from build123d import *

# Parameters (mm, degrees)
SKETCH2_R            = 65
SKETCH2_R_2          = 36
RING_EXTRUSION_DEPTH = 2
GROOVES_DEPTH        = 1
CIRPATTERN2_COUNT    = 12
FILLET3_R            = 0.5


with BuildPart() as part:
    # Sketch2 → ring extrusion (new body)
    with BuildSketch(Plane(origin=(0, 0, 0), x_dir=(1, 0, 0), z_dir=(0, 1, 0))):
        with Locations(Location((0, 0, 0), (0, 0, 270))):
            Circle(SKETCH2_R)
        with Locations(Location((0, 0, 0), (0, 0, 270))):
            Circle(SKETCH2_R_2, mode=Mode.SUBTRACT)
    extrude(amount=RING_EXTRUSION_DEPTH)

    # Sketch5 → grooves (cut)
    with BuildSketch(Plane(origin=(0, 2, 0), x_dir=(1, 0, 0), z_dir=(0, 1, 0))):
        with BuildLine():
            Line((-43, 38.6), (7, 38.6))
            ThreePointArc((7, 38.6), (7.6, 38), (7, 37.4))
            Line((7, 37.4), (-43, 37.4))
            ThreePointArc((-43, 37.4), (-43.6, 38), (-43, 38.6))
        make_face()
    grooves = extrude(amount=-GROOVES_DEPTH, mode=Mode.SUBTRACT)

    # CirPattern2: grooves ×12 about axis
    cirpattern2_axis = Axis((0, 0, 0), (0, 1, 0))
    for i in range(1, CIRPATTERN2_COUNT):
        add(grooves.rotate(cirpattern2_axis, i * 360 / CIRPATTERN2_COUNT), mode=Mode.SUBTRACT)

    # Fillet3
    fillet3_edges = [part.edges().sort_by_distance(p)[0] for p in [
        (0, 0, -65),
        (0, 2, -65),
        (0, 0, -36),
        (0, 2, -36),
    ]]
    fillet(fillet3_edges, radius=FILLET3_R)


solid = part.part
For this review, take the finished solid that the model builds, in its own axes (mm). A direction names the side the tool comes from. Round coordinates to 2 decimals unless told otherwise and drop trailing zeros. One line per item, written item: value. Start each with the question number.
Item 1: Clearance check with flat-ended pins moving along their axes: pin 1 Ø0.5 at (y, z) = (1.5, -28.5) entering from +X; pin 2 Ø1 at (y, z) = (1.5, 23.5) entering from +X; pin 3 Ø1.1 at (y, z) = (1.5, 10.5) entering from -X. State where each tip first meets the part, or that it passes through.
Item 2: The part is to be moulded in two halves that separate along Z. For faces 1 (the cylindrical face through (19.52, 0.99, 62)), 2 (the flat face through (-42, 2, -1)), 3 (the flat face through (34, 1, 24)), say which applies: +Z half, -Z half, draft (parallel to the pull), parting line (faces both ways), or undercut.
Item 3: For L1, parallel to Z at x = 50.5, y = 1.6; L2, parallel to X at y = 1.55, z = 49.5; L3, parallel to Z at x = 12, y = 1.8, list the stretches that pass through material, from the lowest coordinate up.
Item 4: For faces 4 (the flat face through (-23.56, 1.51, 33.99)), 5 (the cylindrical face through (10.81, 0.99, 34.34)), list the 3-axis set-ups (+Z, -Z, +X, -X, +Y, -Y) from which the entire face can be reached by the end or side of a thin tool; tool diameter is ignored.
Answer below:
1. pin 1: stops at x = 58.54
1. pin 2: stops at x = 60.79
1. pin 3: stops at x = -64.23
2. face 1: parting line
2. face 2: draft
2. face 3: undercut
3. L1: z = -40.91 to -12.67, -10.27 to 14.03, 15.42 to 40.91
3. L2: x = -42.12 to -15.99, -14.61 to 8.54, 10.94 to 42.12
3. L3: z = -63.78 to -56.42, -54.02 to -37.64, -36.26 to -34.05, 34.05 to 37.4, 38.6 to 50.11, 51.5 to 63.78
4. face 4: +Y
4. face 5: +Y, -Y
